from build123d import *

# Parameters (mm, degrees)
F1_DEPTH = 4.2
F2_W     = 20.9
F2_H     = 4.1
F3_DEPTH = 10
F5_DEPTH = 4.1


with BuildPart() as f1:
    # F0 (on Top) → F1 (new body)
    with BuildSketch(Plane.XY):
        with BuildLine():
            Line((0, 7.95), (-8.199971, 7.95))
            Line((-8.199971, 7.95), (-10.55, 5.05))
            Line((-10.55, 5.05), (-10.55, -4.15))
            Line((-10.55, -4.15), (-7.678119, -6.975643))
            ThreePointArc((-7.678119, -6.975643), (-7.033292, -7.400849), (-6.275429, -7.55))
            Line((-6.275429, -7.55), (-6.046804, -7.55))
            ThreePointArc((-6.046804, -7.55), (-5.653998, -7.511047), (-5.276493, -7.395704))
            Line((-5.276493, -7.395704), (-1.155466, -5.675779))
            ThreePointArc((-1.155466, -5.675779), (0, -5.444335), (1.155466, -5.675779))
            Line((1.155466, -5.675779), (5.276493, -7.395704))
            ThreePointArc((5.276493, -7.395704), (5.653998, -7.511047), (6.046804, -7.55))
            Line((6.046804, -7.55), (6.275429, -7.55))
            ThreePointArc((6.275429, -7.55), (7.033292, -7.400849), (7.678119, -6.975643))
            Line((7.678119, -6.975643), (10.55, -4.15))
            Line((10.55, -4.15), (10.55, 5.05))
            Line((10.55, 5.05), (8.199971, 7.95))
            Line((8.199971, 7.95), (0, 7.95))
        make_face()
    extrude(amount=F1_DEPTH)

    # F2 (on face) → F3 (cut)
    with BuildSketch(Plane.XZ.offset(7.55)):
        with Locations((0, 2.05)):
            Rectangle(F2_W, F2_H)
    extrude(amount=-F3_DEPTH, mode=Mode.SUBTRACT)

    # F4 (on face) → F5 (cut)
    with BuildSketch(Plane(origin=(0, 0, 0), x_dir=(1, 0, 0), z_dir=(0, 0, -1))):
        Polygon((10.45, -2.45), (-10.45, -2.45), (-10.45, -5.05), (-7.217863, -9.038545), (7.210609, -9.047497), (10.45, -5.05), align=None)
    extrude(amount=-F5_DEPTH, mode=Mode.SUBTRACT)


solid = f1.part
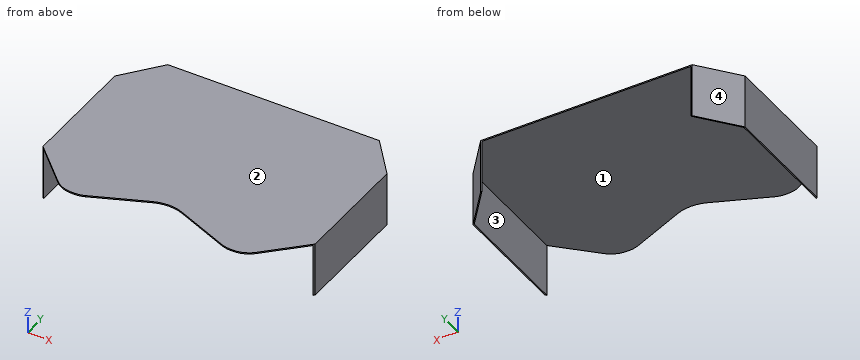
Here's how the part is built. I have some questions about the finished solid (model axes, mm). Face numbers are marked on the shaded views. Coordinates: 2 decimals unless noted, no trailing zeros. Order: outer loops, then holes, each group sorted by start corner. A loop starts at its lowest first (then second) coordinate and runs counter-clockwise, first axis right, second up. Notation, with made-up numbers: M 45,-19 L 69,-19 A12 cw 69,2 Z; hole C 25,74 d5. An arc over 180 degrees is marked long. Answer as CSV lines item,"result". Start each with the question number.
1. I want a section at C-C, the plane x = 8.75. Write out the boundary of the cut face in (y, z).
2. For pin 1 (4 mm diameter, centred on x = -4.5, y = -2, fed in from -Z), with a flat end and sliding along its axis, tell me the tip position at first contact or that it passes through.
3. I want a section at D-D, the plane y = 6. Write out the boundary of the cut face in (x, z).
4. We'd pull the mould along X, two halves only. Please class the marked faces 1, 2, 3 and 4: released by +X, released by -X, zero draft, split by the parting line, or undercut.
5. I want a section at B-B, the plane y = -2. Write out the boundary of the cut face in (x, z), and give its area (3 significant figures).
6. I want a section at A-A, the plane z = 0.9. Write out the boundary of the cut face in (x, y).
Recorded:
1,outline,"M -5.92,4.1 L 7.15,4.1 L 7.15,0 L 7.27,0 L 7.27,4.2 L -5.92,4.2 Z"
2,pin 1,"stops at z = 4.1"
3,outline,"M -9.78,0 L -9.68,0 L -9.68,4.1 L 9.68,4.1 L 9.68,0 L 9.78,0 L 9.78,4.2 L -9.78,4.2 Z"
4,face 1,"undercut"
4,face 2,"zero draft"
4,face 3,"undercut"
4,face 4,"released by -X"
5,outline,"M -10.55,0 L -10.45,0 L -10.45,4.1 L 10.45,4.1 L 10.45,0 L 10.55,0 L 10.55,4.2 L -10.55,4.2 Z"
5,area,"2.93 mm2"
6,outline,"M -10.55,-4.15 L -10.45,-4.25 L -10.45,5.05 L -8.1,7.95 L -8.2,7.95 L -10.55,5.05 Z; M 8.1,7.95 L 10.45,5.05 L 10.45,-4.25 L 10.55,-4.15 L 10.55,5.05 L 8.2,7.95 Z"
